Here's the drawing with two shaded views (mm, measured from the low corner). I have some questions. Give positions to 0.01 mm unless a question says otherwise; leave off trailing zeros. Answer as CSV lines item,"result". Start each with the question number.
Q1. If I drill on line 1 along X through (y, z) = (2.35, 7.5) (1 decimal); line 2 along X through (y, z) = (1.35, 6.35); line 3 along Z through (x, y) = (4.5, 2.25) (1 decimal), over which ranges is the centre line in solid material (lowest first)?
Q2. Imagine slicing it at A-A on z = 6.35. State how many separate pieces and enclosed holes the cut face has, and give its area (3 significant figures).
Q3. Will these pins go through, and if not, where does the flat tip stop? pin 1 Ø2 at (x, z) = (38.1, 44.15) entering from +Y; pin 2 Ø3.5 at (x, z) = (38.1, 6.35) entering from +Y; pin 3 Ø1.5 at (y, z) = (2.5, 32.5) entering from -X (1 decimal).
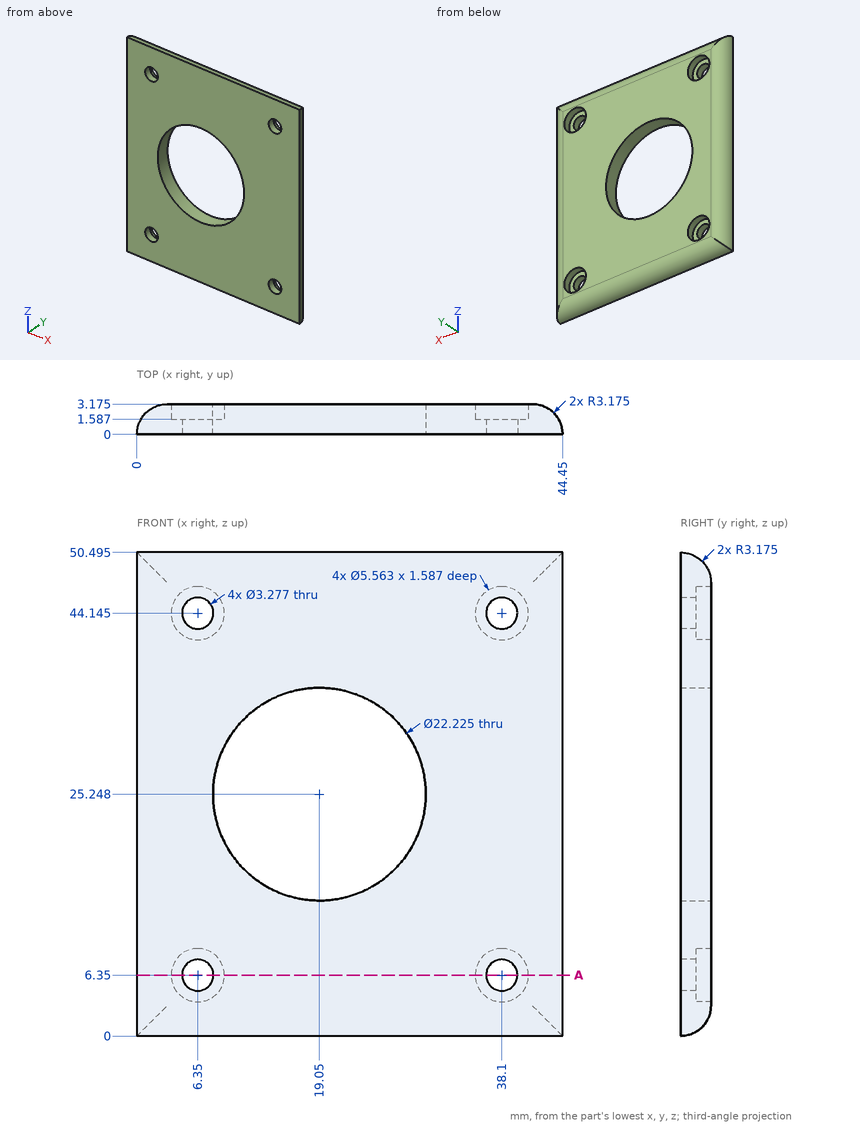
Conclusion:
1,line 1,"1 to 3.8, 8.9 to 35.6, 40.6 to 43.4"
1,line 2,"0.3 to 4.71, 7.99 to 36.46, 39.74 to 44.15"
1,line 3,"0.9 to 4.3, 8.4 to 42.1, 46.2 to 49.6"
2,separate pieces,"3"
2,enclosed holes,"0"
2,area,"109 mm^2"
3,pin 1,"through"
3,pin 2,"y = 1.59"
3,pin 3,"x = 0.5"
